from build123d import *

# Parameters (mm, degrees)
SKETCH2_R          = 8
SKETCH2_R_2        = 1.25
CUT_EXTRUDE1_DEPTH = 15


with BuildPart() as part:
    # Sketch1 → Revolve1 (revolve)
    with BuildSketch(Plane.XY):
        Polygon((0, 10.150862069), (24, 10.150862069), (24, 15.150862069), (31, 15.150862069), (31, 14.650862069), (30, 14.650862069), (30, -0.349137931), (31, -0.349137931), (31, -0.849137931), (24, -0.849137931), (24, 4.150862069), (0, 4.150862069), align=None)
    revolve(axis=Axis((0, 36.012931034, 0), (0, -1, 0)))

    # Sketch2 → Cut-Extrude1 (cut, symmetric)
    with BuildSketch(Plane(origin=(0, 10.150862069, 0), x_dir=(1, 0, 0), z_dir=(0, 1, 0))):
        Circle(SKETCH2_R)
        with Locations((11, 0)):
            Circle(SKETCH2_R_2)
        with Locations((5.5, -9.526279442)):
            Circle(SKETCH2_R_2)
        with Locations((-5.5, -9.526279442)):
            Circle(SKETCH2_R_2)
        with Locations((-11, 0)):
            Circle(SKETCH2_R_2)
        with Locations((-5.5, 9.526279442)):
            Circle(SKETCH2_R_2)
        with Locations((5.5, 9.526279442)):
            Circle(SKETCH2_R_2)
    extrude(amount=CUT_EXTRUDE1_DEPTH, both=True, mode=Mode.SUBTRACT)


solid = part.part
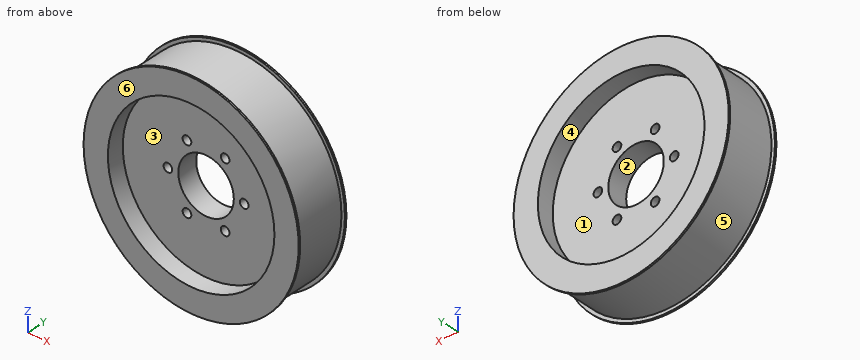
Here's how the part is built. I have some questions about the finished solid (model axes, mm). Face numbers are marked on the shaded views. A direction names the side the tool comes from. Round coordinates to 2 decimals unless told otherwise and drop trailing zeros. Order: outer loops, then holes, each group sorted by start corner. A loop starts at its lowest first (then second) coordinate and runs counter-clockwise, first axis right, second up. Notation, with made-up numbers: (40, 20) -> (83, 20) arc R19 ccw to (83, 54) -> close; hole circle Ø7 at (-40, 16). An arc over 180 degrees is marked (long way). Return JSON: item names as keys, results as strings.
Q1. If we section it at D-D on y = 5.75: List the corners of the cut face in (x, z) for me, plus the area to 3 significant figures.
Filled sheet:
{"outline": "circle Ø60 at (0, 0); hole circle Ø2.5 at (-11, 0); hole circle Ø16 at (0, 0); hole circle Ø2.5 at (-5.5, -9.53); hole circle Ø2.5 at (-5.5, 9.53); hole circle Ø2.5 at (5.5, -9.53); hole circle Ø2.5 at (5.5, 9.53); hole circle Ø2.5 at (11, 0)", "area": "2,600 mm^2"}
Q2. If we mould it in two halves opening along Z, with no side actions, what happens to the marked faces 4, 5 and 6? For each: released by +Z, released by -Z, zero draft, split by the parting line, or undercut.
Filled sheet:
{"face 4": "undercut", "face 5": "split by the parting line", "face 6": "zero draft"}
Q3. If we section it at A-A on x = 0: List the corners of the cut face in (y, z) for me.
Filled sheet:
{"outline": "(-0.85, -31) -> (-0.35, -31) -> (-0.35, -30) -> (14.65, -30) -> (14.65, -31) -> (15.15, -31) -> (15.15, -24) -> (10.15, -24) -> (10.15, -8) -> (4.15, -8) -> (4.15, -24) -> (-0.85, -24) -> close; (-0.85, 24) -> (4.15, 24) -> (4.15, 8) -> (10.15, 8) -> (10.15, 24) -> (15.15, 24) -> (15.15, 31) -> (14.65, 31) -> (14.65, 30) -> (-0.35, 30) -> (-0.35, 31) -> (-0.85, 31) -> close"}
Q4. For pin 1 Ø3 at (x, z) = (5.5, -9.53) entering from -Y; pin 2 Ø3 at (x, z) = (-5.5, -9.53) entering from +Y; pin 3 Ø6 at (x, y) = (12, 6.5) entering from +Z, each with a flat end and sliding along its axis, tell me the tip position at first contact or that it passes through.
Filled sheet:
{"pin 1": "stops at y = 4.15", "pin 2": "stops at y = 10.15", "pin 3": "stops at z = 28.62"}
Q5. If we section it at B-B on z = -4: List the corners of the cut face in (x, y) for me.
Filled sheet:
{"outline": "(-30.74, -0.85) -> (-23.66, -0.85) -> (-23.66, 4.15) -> (-6.93, 4.15) -> (-6.93, 10.15) -> (-23.66, 10.15) -> (-23.66, 15.15) -> (-30.74, 15.15) -> (-30.74, 14.65) -> (-29.73, 14.65) -> (-29.73, -0.35) -> (-30.74, -0.35) -> close; (6.93, 4.15) -> (23.66, 4.15) -> (23.66, -0.85) -> (30.74, -0.85) -> (30.74, -0.35) -> (29.73, -0.35) -> (29.73, 14.65) -> (30.74, 14.65) -> (30.74, 15.15) -> (23.66, 15.15) -> (23.66, 10.15) -> (6.93, 10.15) -> close"}
Q6. Which directions (+Z, -Z, +X, -X, +Y, -Y) give clear straight access to the entire face, cutting with the end or side of a thin tool? Please do the marked faces 1, 2 and 3.
Filled sheet:
{"face 1": "+Y", "face 2": "+Y, -Y", "face 3": "-Y"}
Q7. If we section it at C-C on z = -13: List the corners of the cut face in (x, y) for me.
Filled sheet:
{"outline": "(-28.14, -0.85) -> (-20.17, -0.85) -> (-20.17, 4.15) -> (20.17, 4.15) -> (20.17, -0.85) -> (28.14, -0.85) -> (28.14, -0.35) -> (27.04, -0.35) -> (27.04, 14.65) -> (28.14, 14.65) -> (28.14, 15.15) -> (20.17, 15.15) -> (20.17, 10.15) -> (-20.17, 10.15) -> (-20.17, 15.15) -> (-28.14, 15.15) -> (-28.14, 14.65) -> (-27.04, 14.65) -> (-27.04, -0.35) -> (-28.14, -0.35) -> close"}
Q8. I need wall thicknesses on line 1 along Z through (x, y) = (5.5, 6.5); line 2 along Z through (x, y) = (0, 2.2); line 3 along Y through (x, z) = (12.5, 5). Which ranges of each line are inside material? Lowest first, please. Write a range as from..to.
Filled sheet:
{"line 1": "z = -29.49..-10.78, -8.28..-5.81, 5.81..8.28, 10.78..29.49", "line 2": "z = -30..-24, 24..30", "line 3": "y = 4.15..10.15"}
